```python
from build123d import *

# Parameters (mm, degrees)
CROQUIS1_W              = 55
CROQUIS1_H              = 35
SALIENTE_EXTRUIR1_DEPTH = 100
CROQUIS2_R              = 4
CORTAR_EXTRUIR1_DEPTH   = 100
CROQUIS3_W              = 35
CROQUIS3_H              = 55
CORTAR_EXTRUIR2_DEPTH   = 39
CROQUIS6_W              = 20
CROQUIS6_H              = 4
CORTAR_EXTRUIR3_DEPTH   = 55
CROQUIS7_R              = 4.05
CORTAR_EXTRUIR4_DEPTH   = 55
REDONDEO1_R             = 10
REDONDEO2_R             = 10
CROQUIS8_R              = 1.6
CORTAR_EXTRUIR5_DEPTH   = 20


with BuildPart() as part:
    # Croquis1 → Saliente-Extruir1 (new body)
    with BuildSketch(Plane.XY):
        Rectangle(CROQUIS1_W, CROQUIS1_H)
    extrude(amount=SALIENTE_EXTRUIR1_DEPTH)

    # Croquis2 → Cortar-Extruir1 (cut)
    with BuildSketch(Plane(origin=(27.5, 0, 0), x_dir=(0, 0, -1), z_dir=(1, 0, 0))):
        with Locations(Location((-82.5, 0, 0), (0, 0, 90))):
            Circle(CROQUIS2_R)
        with BuildLine():
            ThreePointArc((-100, 0), (-94.874368671, 12.374368671), (-82.5, 17.5))
            Line((-82.5, 17.5), (-100, 17.5))
            Line((-100, 17.5), (-100, 0))
        make_face()
        with BuildLine():
            ThreePointArc((-82.5, -17.5), (-94.874368671, -12.374368671), (-100, 0))
            Line((-100, 0), (-100, -17.5))
            Line((-100, -17.5), (-82.5, -17.5))
        make_face()
    extrude(amount=-CORTAR_EXTRUIR1_DEPTH, mode=Mode.SUBTRACT)

    # Croquis3 → Cortar-Extruir2 (cut)
    with BuildSketch(Plane(origin=(0, 17.5, 0), x_dir=(1, 0, 0), z_dir=(0, 1, 0))):
        with Locations((0, -72.5)):
            Rectangle(CROQUIS3_W, CROQUIS3_H)
    extrude(amount=-CORTAR_EXTRUIR2_DEPTH, mode=Mode.SUBTRACT)

    # Croquis6 → Cortar-Extruir3 (cut)
    with BuildSketch(Plane(origin=(27.5, 0, 0), x_dir=(0, 0, -1), z_dir=(1, 0, 0))):
        Polygon((-45, 17.5), (0, 17.5), (0, 10), (-20, 10), align=None)
        with Locations((-10, 0)):
            Rectangle(CROQUIS6_W, CROQUIS6_H)
        Polygon((-45, -17.5), (-20, -10), (0, -10), (0, -17.5), align=None)
    extrude(amount=-CORTAR_EXTRUIR3_DEPTH, mode=Mode.SUBTRACT)

    # Croquis7 → Cortar-Extruir4 (cut)
    with BuildSketch(Plane(origin=(0, 0, 0), x_dir=(-1, 0, 0), z_dir=(0, 0, -1))):
        with Locations((-10, 0)):
            Circle(CROQUIS7_R)
        with Locations((10, 0)):
            Circle(CROQUIS7_R)
    extrude(amount=-CORTAR_EXTRUIR4_DEPTH, mode=Mode.SUBTRACT)

    # Redondeo1
    # the kernel refuses this fillet: 10 mm, written as the material it adds along each edge
    with BuildSketch(Plane(origin=(-17.5, 17.5, 45), x_dir=(1, 0, 0), z_dir=(0, -1, 0))) as redondeo1_piece_1_section:
        with BuildLine():
            CenterArc((REDONDEO1_R, REDONDEO1_R), REDONDEO1_R, 180, 90)
            Line((0, REDONDEO1_R), (0, 0))
            Line((0, 0), (REDONDEO1_R, 0))
        make_face()
    redondeo1_piece_1 = extrude(amount=35, mode=Mode.PRIVATE)
    redondeo1_piece_1 = split(redondeo1_piece_1, bisect_by=Plane(origin=(-15.390656306, -16.700081338, 42.33360446), z_dir=(0, 0.9578262852211515, 0.2873478855663453)), keep=Keep.TOP, mode=Mode.PRIVATE)
    redondeo1_piece_1 = split(redondeo1_piece_1, bisect_by=Plane(origin=(-15.390656306, 16.700081275, 42.333604252), z_dir=(0, -0.9578262852211514, 0.28734788556634544)), keep=Keep.TOP, mode=Mode.PRIVATE)
    redondeo1_piece_1 = redondeo1_piece_1 - Plane(origin=(-10, 0, 47.343628748), x_dir=(-1, 0, 0), z_dir=(0, 0, -1)) * Cylinder(4.05, 110, mode=Mode.PRIVATE)
    add(redondeo1_piece_1)

    # Redondeo2
    # the kernel refuses this fillet: 10 mm, written as the material it adds along each edge
    with BuildSketch(Plane(origin=(17.5, 17.5, 45), x_dir=(0, 0, 1), z_dir=(0, -1, 0))) as redondeo2_piece_1_section:
        with BuildLine():
            CenterArc((REDONDEO2_R, REDONDEO2_R), REDONDEO2_R, 180, 90)
            Line((0, REDONDEO2_R), (0, 0))
            Line((0, 0), (REDONDEO2_R, 0))
        make_face()
    redondeo2_piece_1 = extrude(amount=35, mode=Mode.PRIVATE)
    redondeo2_piece_1 = redondeo2_piece_1 - Plane(origin=(10, 0, 47.343628624), x_dir=(-1, 0, 0), z_dir=(0, 0, -1)) * Cylinder(4.05, 110, mode=Mode.PRIVATE)
    redondeo2_piece_1 = split(redondeo2_piece_1, bisect_by=Plane(origin=(15.390657599, 16.700081065, 42.333603552), z_dir=(0, -0.9578262852211514, 0.28734788556634544)), keep=Keep.TOP, mode=Mode.PRIVATE)
    redondeo2_piece_1 = split(redondeo2_piece_1, bisect_by=Plane(origin=(15.390657599, -16.70008148, 42.333604932), z_dir=(0, 0.9578262852211515, 0.2873478855663453)), keep=Keep.TOP, mode=Mode.PRIVATE)
    add(redondeo2_piece_1)

    # Croquis8 → Cortar-Extruir5 (cut)
    with BuildSketch(Plane(origin=(0, 10, 0), x_dir=(1, 0, 0), z_dir=(0, 1, 0))):
        with Locations(Location((0, -10, 0), (0, 0, 180))):
            Circle(CROQUIS8_R)
        with Locations(Location((-19.75, -10, 0), (0, 0, 180))):
            Circle(CROQUIS8_R)
        with Locations(Location((19.75, -10, 0), (0, 0, 180))):
            Circle(CROQUIS8_R)
    extrude(amount=-CORTAR_EXTRUIR5_DEPTH, mode=Mode.SUBTRACT)


solid = part.part
```
Can you work these out from the model? Positions are in its coordinate system, mm. A direction names the side the tool comes from. Coordinates: 2 decimals unless noted, no trailing zeros. Order: outer loops, then holes, each group sorted by start corner. A loop starts at its lowest first (then second) coordinate and runs counter-clockwise, first axis right, second up.
1. If we section it at D-D (x = -10): Please give me the cut outline in (y, z).
2. For faces 5 (the face through (0, -2, 12)), 6 (the face through (0, -10, 12)), 7 (the face through (22.57, -0.867, 78.595)), 8 (the face through (-14.65, 0.25, 48.01)), 9 (the face through (0.35, 6.06, 8.44)), which set-ups out of +Z, -Z, +X, -X, +Y, -Y let a thin tool reach every point of the face, with its end or its side?
3. I'm going to push flat-ended pins straight in: pin 1 (16 mm diameter, centred on x = 0.5, z = 11, fed in from +Y); pin 2 (15.5 mm diameter, centred on x = -20.5, z = 12, fed in from -Y); pin 3 (2 mm diameter, centred on x = 22, y = -0.5, fed in from -Z). Where does each tip first touch, or does it pass through?
4. If we section it at B-B (x = 0): Please give me the cut outline in (y, z).
5. I need wall thicknesses on line 1 (X direction, y = 0, z = 28); line 2 (Y direction, x = -18, z = 16.5); line 3 (X direction, y = 5, z = 84.5). Which ranges of each line are inside material? Lowest first, please.
6. If we section it at C-C (y = -8): Please give me the cut outline in (x, z), then the cut area to 3 significant figures.
7. If we section it at A-A (x = 19.75): Please give me the cut outline in (y, z).
8. Thinking about a two-plate mould opening in Y: for faces 1 (the face through (22, -2, 10)), 2 (the face through (14.046, 0.178, 23.39)), 3 (the face through (-17.5, 0, 78)), 4 (the face through (22, -17.5, 64)), which applies, +Y half, -Y half, draft (parallel to the pull), parting line (faces both ways), or undercut?
Entries:
1. outline: (-17.5, 45) - (-10, 20) - (-10, 0) - (-4.05, 0) - (-4.05, 45.32) - (-17.5, 45.32) - close; (4.05, 0) - (10, 0) - (10, 20) - (17.5, 45) - (17.5, 45.32) - (4.05, 45.32) - close
2. face 5: -Z, +X, -X
2. face 6: -Z, +X, -X, -Y
2. face 7: +X, -X
2. face 8: +Z, +Y, -Y
2. face 9: +Y, -Y
3. pin 1: stops at y = 10
3. pin 2: stops at y = -10
3. pin 3: stops at z = 20
4. outline: (-17.5, 45) - (-10, 20) - (-10, 11.6) - (-2, 11.6) - (-2, 20) - (2, 20) - (2, 11.6) - (10, 11.6) - (10, 20) - (17.5, 45) - close; (-10, 0) - (-2, 0) - (-2, 8.4) - (-10, 8.4) - close; (2, 0) - (10, 0) - (10, 8.4) - (2, 8.4) - close
5. line 1: x = -27.5 to -14.05, -5.95 to 5.95, 14.05 to 27.5
5. line 2: y = -10 to -2, 2 to 10
5. line 3: x = -27.5 to -17.5, 17.5 to 27.5
6. outline: (-27.5, 0) - (27.5, 0) - (27.5, 98.06) - (17.5, 98.06) - (17.5, 55) arc R10 cw to (7.5, 45) - (-7.5, 45) arc R10 cw to (-17.5, 55) - (-17.5, 98.06) - (-27.5, 98.06) - close; hole circle Ø3.2 at (-19.75, 10); hole circle Ø3.2 at (0, 10); hole circle Ø3.2 at (19.75, 10)
6. area: 3,560 mm2
7. outline: (-17.5, 45) - (-10, 20) - (-10, 11.6) - (-2, 11.6) - (-2, 20) - (2, 20) - (2, 11.6) - (10, 11.6) - (10, 20) - (17.5, 45) - (17.5, 82.5) arc R17.5 ccw to (-17.5, 82.5) - close; (-10, 0) - (-2, 0) - (-2, 8.4) - (-10, 8.4) - close; (2, 0) - (10, 0) - (10, 8.4) - (2, 8.4) - close; hole circle Ø8 at (0, 82.5)
8. face 1: undercut
8. face 2: undercut
8. face 3: draft
8. face 4: -Y half
